from build123d import *

# Parameters (mm, degrees)
SCHIZZO2_W                   = 42
SCHIZZO2_H                   = 14.5
SCHIZZO2_R                   = 3
SCHIZZO2_R_2                 = 1
ESTRUSIONE_ESTRUSIONE1_DEPTH = 1
SCHIZZO4_W                   = 1
SCHIZZO4_H                   = 5
SCHIZZO4_H_2                 = 4
ESTRUSIONE_ESTRUSIONE2_DEPTH = 2
SCHIZZO5_R                   = 1.5
SCHIZZO5_R_2                 = 1
ESTRUSIONE_ESTRUSIONE3_DEPTH = 1
TAGLIO_ESTRUSIONE1_START     = -1
TAGLIO_ESTRUSIONE1_DEPTH     = 1
ESTRUSIONE_ESTRUSIONE4_START = 1
SCHIZZO7_R                   = 1.5
ESTRUSIONE_ESTRUSIONE4_DEPTH = 1


with BuildPart() as part:
    # Schizzo2 → Estrusione-Estrusione1 (new body)
    with BuildSketch(Plane.XY):
        Rectangle(SCHIZZO2_W, SCHIZZO2_H)
        with Locations((9, 1.25)):
            Circle(SCHIZZO2_R, mode=Mode.SUBTRACT)
        with Locations((-1.2, 2.25)):
            Circle(SCHIZZO2_R_2, mode=Mode.SUBTRACT)
        with Locations((-10, 1.25)):
            Circle(SCHIZZO2_R_2, mode=Mode.SUBTRACT)
    extrude(amount=ESTRUSIONE_ESTRUSIONE1_DEPTH)

    # Schizzo4 → Estrusione-Estrusione2 (add)
    with BuildSketch(Plane.XY.offset(1)):
        with Locations((18, 4.75)):
            Rectangle(SCHIZZO4_W, SCHIZZO4_H)
        with Locations((18, -5.25)):
            Rectangle(SCHIZZO4_W, SCHIZZO4_H_2)
        with Locations((-18, -5.25)):
            Rectangle(SCHIZZO4_W, SCHIZZO4_H_2)
        with Locations((-18, 4.75)):
            Rectangle(SCHIZZO4_W, SCHIZZO4_H)
    extrude(amount=ESTRUSIONE_ESTRUSIONE2_DEPTH)

    # Schizzo5 → Estrusione-Estrusione3 (add)
    # profile 1 of 6: a face of its own
    with BuildSketch(Plane.XY.offset(1)):
        with Locations(Location((-1.2, 2.25, 0), (0, 0, 180))):
            Circle(SCHIZZO5_R)
        with Locations((-1.2, 2.25)):
            Circle(SCHIZZO5_R_2, mode=Mode.SUBTRACT)
    # profile 2 of 6: a face of its own
    with BuildSketch(Plane.XY.offset(1)):
        with Locations(Location((-10, 1.25, 0), (0, 0, 180))):
            Circle(SCHIZZO5_R)
        with Locations((-10, 1.25)):
            Circle(SCHIZZO5_R_2, mode=Mode.SUBTRACT)
    # profile 3 of 6: a face of its own
    with BuildSketch(Plane.XY.offset(1)):
        with BuildLine():
            Line((-17.5, 7.214212601), (-17.5, 5.014576268))
            ThreePointArc((-17.5, 5.014576268), (-15.362109211, 5.114234355), (-15.5, 7.25))
            Line((-15.5, 7.25), (-17.46, 7.25))
            ThreePointArc((-17.46, 7.25), (-17.480160079, 7.232285223), (-17.5, 7.214212601))
        make_face()
        with Locations((-16.48, 6.114394435)):
            Circle(SCHIZZO5_R_2, mode=Mode.SUBTRACT)
    # profile 4 of 6: a face of its own
    with BuildSketch(Plane.XY.offset(1)):
        with BuildLine():
            Line((-17.46, -7.25), (-15.5, -7.25))
            ThreePointArc((-15.5, -7.25), (-15.362109211, -5.114234355), (-17.5, -5.014576268))
            Line((-17.5, -5.014576268), (-17.5, -7.214212601))
            ThreePointArc((-17.5, -7.214212601), (-17.480160079, -7.232285223), (-17.46, -7.25))
        make_face()
        with Locations(Location((-16.48, -6.114394435, 0), (0, 0, 180))):
            Circle(SCHIZZO5_R_2, mode=Mode.SUBTRACT)
    # profile 5 of 6: a face of its own
    with BuildSketch(Plane.XY.offset(1)):
        with BuildLine():
            Line((17.46, -7.25), (15.5, -7.25))
            ThreePointArc((15.5, -7.25), (15.362109211, -5.114234355), (17.5, -5.014576268))
            Line((17.5, -5.014576268), (17.5, -7.214212601))
            ThreePointArc((17.5, -7.214212601), (17.480160079, -7.232285223), (17.46, -7.25))
        make_face()
        with Locations((16.48, -6.114394435)):
            Circle(SCHIZZO5_R_2, mode=Mode.SUBTRACT)
    # profile 6 of 6: a face of its own
    with BuildSketch(Plane.XY.offset(1)):
        with BuildLine():
            Line((17.46, 7.25), (15.5, 7.25))
            ThreePointArc((15.5, 7.25), (15.362109211, 5.114234355), (17.5, 5.014576268))
            Line((17.5, 5.014576268), (17.5, 7.214212601))
            ThreePointArc((17.5, 7.214212601), (17.480160079, 7.232285223), (17.46, 7.25))
        make_face()
        with Locations(Location((16.48, 6.114394435, 0), (0, 0, 180))):
            Circle(SCHIZZO5_R_2, mode=Mode.SUBTRACT)
    extrude(amount=ESTRUSIONE_ESTRUSIONE3_DEPTH)

    # Schizzo6 → Taglio-Estrusione1 (cut)
    with BuildSketch(Plane.XY.offset(2).offset(TAGLIO_ESTRUSIONE1_START)):
        with BuildLine():
            Line((-8.949725473, 2.320945105), (-8.949725473, 0.179054895))
            ThreePointArc((-8.949725473, 0.179054895), (-8.5, 1.25), (-8.949725473, 2.320945105))
        make_face()
    extrude(amount=TAGLIO_ESTRUSIONE1_DEPTH, mode=Mode.SUBTRACT)

    # Schizzo7 → Estrusione-Estrusione4 (add)
    with BuildSketch(Plane(origin=(0, 0, 0), x_dir=(-1, 0, 0), z_dir=(0, 0, -1)).offset(ESTRUSIONE_ESTRUSIONE4_START)):
        with Locations((10, 1.25)):
            Circle(SCHIZZO7_R)
        with BuildLine():
            Line((1.2, 3.75), (1.2, 0.75))
            ThreePointArc((1.2, 0.75), (2.7, 2.25), (1.2, 3.75))
        make_face()
    extrude(amount=-ESTRUSIONE_ESTRUSIONE4_DEPTH)


solid = part.part
Work out the finished part from the listing and answer in its coordinate system (mm). A direction names the side the tool comes from. Give positions to 0.01 mm unless a question says otherwise; leave off trailing zeros. Write each loop counter-clockwise with the first axis right and the second up, starting at its lowest first coordinate (ties: lowest second). Pieces come first, ordered by that corner, then holes.
Q1. Given pin 1 (3 mm diameter, centred on x = 2.5, y = 4.5, fed in from -Z); pin 2 (3 mm diameter, centred on x = 0.5, y = 2.5, fed in from +Z); pin 3 (2 mm diameter, centred on x = 1.5, y = -0.5, fed in from +Z), each flat-ended and moving along its own axis, determine where each tip first touches the part or whether it passes through.
Answer:
pin 1: stops at z = 0
pin 2: stops at z = 2
pin 3: stops at z = 1
Q2. The part is cut by section A-A on x = 9. Give the vertices of the cut face in (y, z), and give its area (3 significant figures).
Answer:
outline: (-7.25, 0) - (-1.75, 0) - (-1.75, 1) - (-7.25, 1) - close; (4.25, 0) - (7.25, 0) - (7.25, 1) - (4.25, 1) - close
area: 8.50 mm2
Q3. The part is cut by section B-B on x = -18. Give the vertices of the cut face in (y, z), and give its area (3 significant figures).
Answer:
outline: (-7.25, 0) - (7.25, 0) - (7.25, 3) - (2.25, 3) - (2.25, 1) - (-3.25, 1) - (-3.25, 3) - (-7.25, 3) - close
area: 32.5 mm2
Q4. For a pull along X with two mould halves and no side action, classify faces 6 (the face through (18.5, -5, 2)), 7 (the face through (-18.5, -5, 2)), 8 (the face through (16, 5, 2)) as released by +X, released by -X, zero draft, split by the parting line, or undercut.
Answer:
face 6: released by +X
face 7: released by -X
face 8: undercut
Q5. The part is cut by section D-D on y = -2.75. Give the vertices of the cut face in (x, z), and give its area (3 significant figures).
Answer:
outline: (-21, 0) - (21, 0) - (21, 1) - (-21, 1) - close
area: 42.0 mm2
Q6. A tool of negligible diameter and unlimited length cuts with its end or side. For faces 1 (the face through (-16, -5, 2)), 2 (the face through (-2, 2, -1)), 3 (the face through (-10.79, 0.64, 0.99)), 4 (the face through (-8.5, 1.3, -0.5)), 5 (the face through (-18, -5, 3)), from which of +Z, -Z, +X, -X, +Y, -Y can it reach the whole face along a straight path? Write none if from no direction.
Answer:
face 1: +Z, +Y, -Y
face 2: -Z, +X, -X, +Y, -Y
face 3: +Z
face 4: -Z
face 5: +Z, +X, -X, +Y, -Y
Q7. The part is cut by section C-C on z = 1.5. State how many separate pieces and enclosed holes the cut face has, and give its area (3 significant figures).
Answer:
separate pieces: 6
enclosed holes: 6
area: 36.0 mm2
Q8. Straight lines are drawn through the part: L1, parallel to X at y = -4.25, z = 2.2; L2, parallel to X at y = -5.5, z = 1.45; L3, parallel to X at y = 2.5, z = 1.05. For each, find the intervals that lie inside material, in ascending order.
Answer:
L1: x = -18.5 to -17.5, 17.5 to 18.5
L2: x = -18.5 to -17.27, -15.69 to -15.11, 15.11 to 15.69, 17.27 to 18.5
L3: x = -18.5 to -17.5, -10.83 to -9.17, -2.68 to -2.17, -0.23 to 0.28, 17.5 to 18.5
